Here's the drawing with two shaded views (mm, measured from the low corner). I have some questions. A direction names the side the tool comes from. Coordinates: 2 decimals unless noted, no trailing zeros. Write each loop counter-clockwise with the first axis right and the second up, starting at its lowest first coordinate (ties: lowest second). Pieces come first, ordered by that corner, then holes. Notation, with made-up numbers: (9, 84.5) - (60, 84.5) arc R16 ccw to (60, 92.5) - close; hole circle Ø11 at (-1, 41.5). An arc over 180 degrees is marked (long way). Answer in a Markdown table with one row per item. Add a question column.
Item 1: Imagine slicing it at C-C (y = 31). Please give me the cut outline in (x, z), plus the area to 3 significant figures.
Item 2: Which directions (+Z, -Z, +X, -X, +Y, -Y) give clear straight access to the entire face, cutting with the end or side of a thin tool? Please do the marked faces 1 and 2.
Item 3: If I drill on probe 1 along Y at (x, z) = (7.5, 9); probe 2 along X at (y, z) = (6.5, 5.25); probe 3 along X at (y, z) = (19.5, 3), over which ranges is the centre line in solid material (lowest first)? Write a range as from..to.
Item 4: Imagine slicing it at B-B (x = 5). Please give me the cut outline in (y, z) (3 decimals), plus the area to 3 significant figures.
Item 5: I'm going to push flat-ended pins straight in: pin 1 (1.5 mm diameter, centred on x = 3.5, y = 17.5, fed in from -Z); pin 2 (3 mm diameter, centred on y = 17.5, z = 7, fed in from -X); pin 3 (1.5 mm diameter, centred on y = 21, z = 1.5, fed in from -X). Where does each tip first touch, or does it pass through?
Item 6: Imagine slicing it at A-A (z = 5). Please give me the cut outline in (x, y) (3 decimals), plus the area to 3 significant figures.
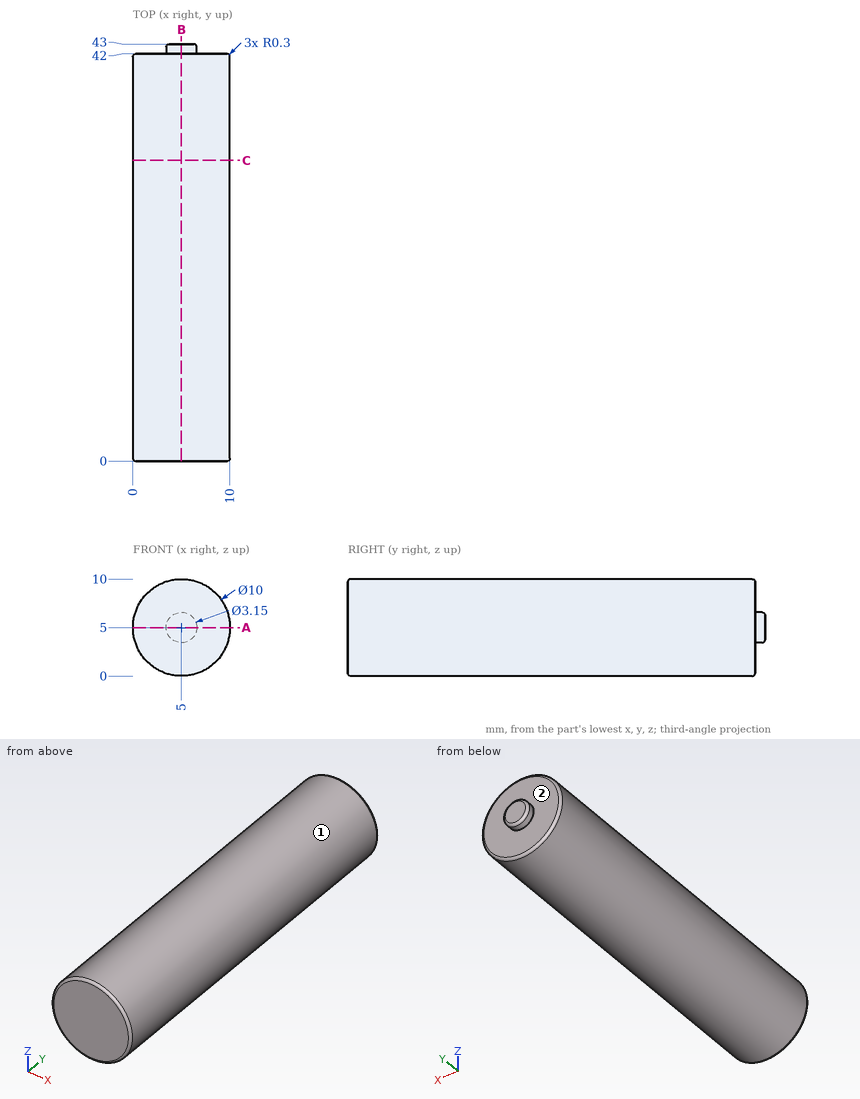
Here are the results:
| question | item | result |
|---|---|---|
| 1 | outline | circle Ø10 at (5, 5) |
| 1 | area | 78.5 mm2 |
| 2 | face 1 | +Y, -Y |
| 2 | face 2 | +Y |
| 3 | probe 1 | y = 0..42 |
| 3 | probe 2 | x = 0.01..9.99 |
| 3 | probe 3 | x = 0.42..9.58 |
| 4 | outline | (0, 0.3) arc R0.3 ccw to (0.3, 0) - (41.7, 0) arc R0.3 ccw to (42, 0.3) - (42, 3.425) - (42.7, 3.425) arc R0.3 ccw to (43, 3.725) - (43, 6.275) arc R0.3 ccw to (42.7, 6.575) - (42, 6.575) - (42, 9.7) arc R0.3 ccw to (41.7, 10) - (0.3, 10) arc R0.3 ccw to (0, 9.7) - close |
| 4 | area | 423 mm2 |
| 5 | pin 1 | stops at z = 0.06 |
| 5 | pin 2 | stops at x = 0.03 |
| 5 | pin 3 | stops at x = 0.82 |
| 6 | outline | (0, 0.3) arc R0.3 ccw to (0.3, 0) - (9.7, 0) arc R0.3 ccw to (10, 0.3) - (10, 41.7) arc R0.3 ccw to (9.7, 42) - (6.575, 42) - (6.575, 42.7) arc R0.3 ccw to (6.275, 43) - (3.725, 43) arc R0.3 ccw to (3.425, 42.7) - (3.425, 42) - (0.3, 42) arc R0.3 ccw to (0, 41.7) - close |
| 6 | area | 423 mm2 |
